Can you work these out from the model? Positions are in its coordinate system, mm. A direction names the side the tool comes from. Give positions to 0.01 mm unless a question says otherwise; leave off trailing zeros. Loops run counter-clockwise (first coordinate to the right, second up) from the corner with the lowest first, then second, coordinate; pieces in that order, holes last. Notation, with made-up numbers: M 38,60.5 L 53,60.5 A14 cw 53,69.5 Z; hole C -14,-19.75 d2. An arc over 180 degrees is marked long. Answer as a JSON object with one key per item and string values.
```python
from build123d import *
from build123d import SkipClean  # not in build123d's __all__

# Parameters (mm, degrees)
F0_R     = 22.225
F1_DEPTH = 33.3248
F0_R_2   = 12.7
F2_DEPTH = 52.3748
F3_DEPTH = 28.575
F4_DEPTH = 20.6248
F5_DEPTH = 3.175
F6_DEPTH = 11.0998
F7_ANGLE = 90


with BuildPart() as f1:
    # F0 (on Top) → F1 (new body)
    with BuildSketch(Plane.XY):
        with BuildLine():
            ThreePointArc((20.32, 15.24), (9.1294627068, 23.7025929106), (-4.8465484826, 24.9333304596))
            ThreePointArc((-4.8465484826, 24.9333304596), (-21.5251259118, -13.4843967044), (20.32, -15.24))
            ThreePointArc((20.32, -15.24), (24.0965557705, -8.0321852568), (25.4, 0))
            ThreePointArc((25.4, 0), (24.0965557705, 8.0321852568), (20.32, 15.24))
        make_face()
        Circle(F0_R, mode=Mode.SUBTRACT)
    extrude(amount=F1_DEPTH)

    # F0 (on Top) → F2 (join)
    with BuildSketch(Plane.XY):
        Circle(F0_R)
        Circle(F0_R_2, mode=Mode.SUBTRACT)
    extrude(amount=F2_DEPTH)

    # F0 (on Top) → F3 (join)
    with BuildSketch(Plane.XY):
        with BuildLine():
            ThreePointArc((123.8244974665, -28.2222222222), (126.1134026015, 14.9803098855), (113.7674148927, 56.4444444444))
            ThreePointArc((113.7674148927, 56.4444444444), (98.7718041015, 62.9734869687), (89.7780268905, 49.313007081))
            ThreePointArc((89.7780268905, 49.313007081), (90.2171864347, 47.1811306981), (91.0139319141, 45.1555555556))
            ThreePointArc((91.0139319141, 45.1555555556), (96.0863854596, 33.0146411355), (99.5472631467, 20.32))
            ThreePointArc((99.5472631467, 20.32), (98.2442480497, 15.0339073716), (93.3255592, 12.7))
            Line((93.3255592, 12.7), (57.15, 12.7))
            Line((57.15, 12.7), (25.4, 12.7))
            ThreePointArc((25.4, 12.7), (22.5601936686, 13.3703873372), (20.32, 15.24))
            ThreePointArc((20.32, 15.24), (24.0965557705, 8.0321852568), (25.4, 0))
            ThreePointArc((25.4, 0), (24.0965557705, -8.0321852568), (20.32, -15.24))
            ThreePointArc((20.32, -15.24), (22.5601936686, -13.3703873372), (25.4, -12.7))
            Line((25.4, -12.7), (54.6792037785, -12.7))
            Line((54.6792037785, -12.7), (93.3255592, -12.7))
            ThreePointArc((93.3255592, -12.7), (98.2442480497, -15.0339073716), (99.5472631467, -20.32))
            ThreePointArc((99.5472631467, -20.32), (99.3098469997, -21.4502747977), (99.0595979732, -22.5777777778))
            ThreePointArc((99.0595979732, -22.5777777778), (108.6198254977, -37.7824497467), (123.8244974665, -28.2222222222))
        make_face()
        with BuildLine():
            ThreePointArc((82.55, 5.5499), (88.0999, 0), (82.55, -5.5499))
            Line((82.55, -5.5499), (44.45, -5.5499))
            ThreePointArc((44.45, -5.5499), (38.9001, 0), (44.45, 5.5499))
            Line((44.45, 5.5499), (82.55, 5.5499))
        make_face(mode=Mode.SUBTRACT)
        with BuildLine():
            ThreePointArc((117.6332725932, -26.8111111111), (110.0309366088, -31.5912248733), (105.2508228466, -23.9888888889))
            ThreePointArc((105.2508228466, -23.9888888889), (107.1963922113, 12.7332634026), (96.7023026588, 47.9777777778))
            ThreePointArc((96.7023026588, 47.9777777778), (99.5684511812, 56.4883707446), (108.079044148, 53.6222222222))
            ThreePointArc((108.079044148, 53.6222222222), (119.8077324715, 14.2312943912), (117.6332725932, -26.8111111111))
        make_face(mode=Mode.SUBTRACT)
    extrude(amount=F3_DEPTH)

    # F0 (on Top) → F4 (join)
    with BuildSketch(Plane.XY):
        with BuildLine():
            ThreePointArc((91.0139319141, 45.1555555556), (90.2171864347, 47.1811306981), (89.7780268905, 49.313007081))
            ThreePointArc((89.7780268905, 49.313007081), (88.599955582, 44.8247099647), (84.6833407547, 42.3361780066))
            Line((84.6833407547, 42.3361780066), (-4.8465484826, 24.9333304596))
            ThreePointArc((-4.8465484826, 24.9333304596), (9.1294627068, 23.7025929106), (20.32, 15.24))
            ThreePointArc((20.32, 15.24), (22.5601936686, 13.3703873372), (25.4, 12.7))
            Line((25.4, 12.7), (57.15, 12.7))
            Line((57.15, 12.7), (93.3255592, 12.7))
            ThreePointArc((93.3255592, 12.7), (98.2442480497, 15.0339073716), (99.5472631467, 20.32))
            ThreePointArc((99.5472631467, 20.32), (96.0863854596, 33.0146411355), (91.0139319141, 45.1555555556))
        make_face()
    extrude(amount=F4_DEPTH)

    # F0 (on Top) → F5 (cut)
    with BuildSketch(Plane.XY):
        with BuildLine():
            ThreePointArc((123.8244974665, -28.2222222222), (126.1134026015, 14.9803098855), (113.7674148927, 56.4444444444))
            ThreePointArc((113.7674148927, 56.4444444444), (98.7718041015, 62.9734869687), (89.7780268905, 49.313007081))
            ThreePointArc((89.7780268905, 49.313007081), (90.2171864347, 47.1811306981), (91.0139319141, 45.1555555556))
            ThreePointArc((91.0139319141, 45.1555555556), (96.0863854596, 33.0146411355), (99.5472631467, 20.32))
            ThreePointArc((99.5472631467, 20.32), (98.2442480497, 15.0339073716), (93.3255592, 12.7))
            Line((93.3255592, 12.7), (57.15, 12.7))
            Line((57.15, 12.7), (25.4, 12.7))
            ThreePointArc((25.4, 12.7), (22.5601936686, 13.3703873372), (20.32, 15.24))
            ThreePointArc((20.32, 15.24), (24.0965557705, 8.0321852568), (25.4, 0))
            ThreePointArc((25.4, 0), (24.0965557705, -8.0321852568), (20.32, -15.24))
            ThreePointArc((20.32, -15.24), (22.5601936686, -13.3703873372), (25.4, -12.7))
            Line((25.4, -12.7), (54.6792037785, -12.7))
            Line((54.6792037785, -12.7), (93.3255592, -12.7))
            ThreePointArc((93.3255592, -12.7), (98.2442480497, -15.0339073716), (99.5472631467, -20.32))
            ThreePointArc((99.5472631467, -20.32), (99.3098469997, -21.4502747977), (99.0595979732, -22.5777777778))
            ThreePointArc((99.0595979732, -22.5777777778), (108.6198254977, -37.7824497467), (123.8244974665, -28.2222222222))
        make_face()
        with BuildLine():
            ThreePointArc((82.55, 5.5499), (88.0999, 0), (82.55, -5.5499))
            Line((82.55, -5.5499), (44.45, -5.5499))
            ThreePointArc((44.45, -5.5499), (38.9001, 0), (44.45, 5.5499))
            Line((44.45, 5.5499), (82.55, 5.5499))
        make_face(mode=Mode.SUBTRACT)
        with BuildLine():
            ThreePointArc((117.6332725932, -26.8111111111), (110.0309366088, -31.5912248733), (105.2508228466, -23.9888888889))
            ThreePointArc((105.2508228466, -23.9888888889), (107.1963922113, 12.7332634026), (96.7023026588, 47.9777777778))
            ThreePointArc((96.7023026588, 47.9777777778), (99.5684511812, 56.4883707446), (108.079044148, 53.6222222222))
            ThreePointArc((108.079044148, 53.6222222222), (119.8077324715, 14.2312943912), (117.6332725932, -26.8111111111))
        make_face(mode=Mode.SUBTRACT)
    with SkipClean():  # cleaning this boolean's faces spoils the solid; the shape is the same uncleaned
        extrude(amount=F5_DEPTH, mode=Mode.SUBTRACT)

    # F0 (on Top) → F6 (cut)
    with BuildSketch(Plane.XY):
        with BuildLine():
            ThreePointArc((91.0139319141, 45.1555555556), (90.2171864347, 47.1811306981), (89.7780268905, 49.313007081))
            ThreePointArc((89.7780268905, 49.313007081), (88.599955582, 44.8247099647), (84.6833407547, 42.3361780066))
            Line((84.6833407547, 42.3361780066), (-4.8465484826, 24.9333304596))
            ThreePointArc((-4.8465484826, 24.9333304596), (9.1294627068, 23.7025929106), (20.32, 15.24))
            ThreePointArc((20.32, 15.24), (22.5601936686, 13.3703873372), (25.4, 12.7))
            Line((25.4, 12.7), (57.15, 12.7))
            Line((57.15, 12.7), (93.3255592, 12.7))
            ThreePointArc((93.3255592, 12.7), (98.2442480497, 15.0339073716), (99.5472631467, 20.32))
            ThreePointArc((99.5472631467, 20.32), (96.0863854596, 33.0146411355), (91.0139319141, 45.1555555556))
        make_face()
    with SkipClean():  # cleaning this boolean's faces spoils the solid; the shape is the same uncleaned
        extrude(amount=F6_DEPTH, mode=Mode.SUBTRACT)


with BuildPart() as f1_1:
    # F7: moved
    add(f1.part.rotate(Axis((59.3627796, 12.7, 28.575), (1, 0, 0)), F7_ANGLE), clean=False)


solid = f1_1.part
```
1) Suppose I cut it at D-D, the plane z = -14. Write out the boundary of the cut face in (x, y), and give its area (3 significant figures).
Answer list:
{"outline": "M 99.56,12.7 L 106.94,12.7 L 106.94,38.1 L 99.56,38.1 Z; M 115.95,12.7 L 123.33,12.7 L 123.33,38.1 L 115.95,38.1 Z", "area": "375 mm^2"}
2) Suppose I cut it at C-C, the plane x = 9. Write out the boundary of the cut face in (y, z) (3 decimals), and give its area (3 significant figures).
Answer list:
{"outline": "M -11.1,-4.446 L 7.95,-4.446 L 7.95,-7.877 L 41.275,-7.877 L 41.275,6.915 L -11.1,6.915 Z; M -11.1,24.835 L 41.275,24.835 L 41.275,39.627 L 30.175,39.627 L 30.175,43.5 L 20.65,43.5 L 20.65,39.627 L 7.95,39.627 L 7.95,36.196 L -11.1,36.196 Z", "area": "1,460 mm^2"}
3) Will these pins go through, and if not, where does the flat tip stop? pin 1 Ø11 at (x, z) = (25.5, 48) entering from +Y; pin 2 Ø5 at (x, z) = (106, 3) entering from +Y; pin 3 Ø8 at (x, y) = (-9.5, 32) entering from +Z.
Answer list:
{"pin 1": "y = 30.18", "pin 2": "y = 38.1", "pin 3": "z = 40.67"}
4) Suppose I cut it at B-B, the plane z = 5. Write out the boundary of the cut face in (x, y) (3 decimals), and give its area (3 significant figures).
Answer list:
{"outline": "M -22.954,7.95 L -19.383,7.95 L -19.383,-11.1 L -6.559,-11.1 L -6.559,41.275 L -22.954,41.275 Z; M 6.559,-11.1 L 19.383,-11.1 L 19.383,7.95 L 22.954,7.95 L 22.954,12.7 L 107.401,12.7 L 107.401,38.1 L 22.954,38.1 L 22.954,41.275 L 6.559,41.275 Z; M 120.159,12.7 L 126.534,12.7 L 126.534,38.1 L 120.159,38.1 Z", "area": "3,890 mm^2"}
5) Please list where these lines run through material, in increasing order: line 1 along Z through (x, y) = (0, 4) (3 decimals); line 2 along Z through (x, y) = (0, 15) (3 decimals); line 3 along X through (y, z) = (14.5, 25). Write a range as from..to.
Answer list:
{"line 1": "-6.35..3.175, 28.575..38.1", "line 2": "-9.525..3.175, 28.575..41.275", "line 3": "-23.7..-8.83, 8.83..107.56, 120.3..126.67"}
6) Suppose I cut it at A-A, the plane y = 9.5. Write out the boundary of the cut face in (x, z) (3 decimals).
Answer list:
{"outline": "C 0,15.875 d50.8; hole C 0,15.875 d25.4"}
7) For faces 1 (the cylindrical face through (38.9, 25.6, 15.8)), 2 (the flat face through (58, 20.65, 43)), 3 (the flat face through (58, 30.175, 43)), which set-ups out of +Z, -Z, +X, -X, +Y, -Y let a thin tool reach every point of the face, with its end or its side?
Answer list:
{"face 1": "+Y, -Y", "face 2": "-Y", "face 3": "+Y"}
8) If we mould it in two halves opening along X, with no side actions, what happens to faces 4 (the cylindrical face through (98.194, 34.193, 30.848)), 5 (the cylindrical face through (-2.89, -1.44, 37.91)), 6 (the flat face through (85, 38.1, 25))? For each: +X half, -X half, draft (parallel to the pull), parting line (faces both ways), or undercut.
Answer list:
{"face 4": "undercut", "face 5": "parting line", "face 6": "draft"}
